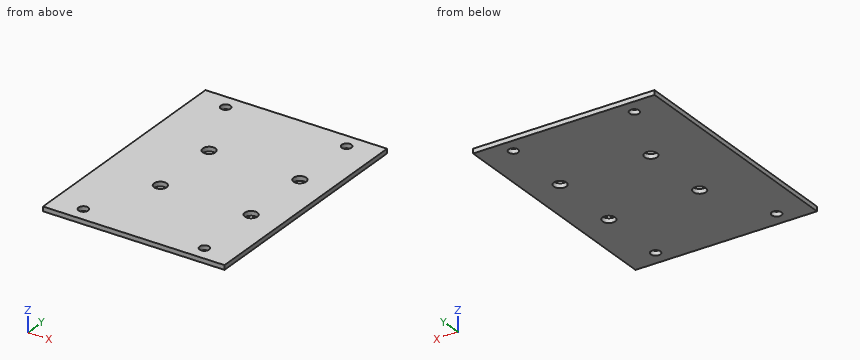
Autodesk Inventor part; units mm, degrees
ref_plane "YZ Plane" through (0, 0, 0) normal (1, 0, 0) x (0, 1, 0)
ref_plane "XZ Plane" through (0, 0, 0) normal (0, 1, 0) x (-1, 0, 0)
ref_plane "XY Plane" through (0, 0, 0) normal (0, 0, 1) x (1, 0, 0)
sketch "スケッチ1" plane through (0, 0, 0) normal (0, 0, 1) x (1, 0, 0)
  line L0 (0, 0) -> (60, 0)
  line L1 (60, 0) -> (60, 80)
  line L2 (60, 80) -> (0, 80)
  line L3 (0, 80) -> (0, 0)
  dimension "d0" = 80
  dimension "d1" = 60
extrude "押し出し1" add sketch "スケッチ1" along normal blind 1.5
sketch "スケッチ2" plane through (0, 0, 1.5) normal (0, 0, 1) x (1, 0, 0)
  line L0 (60, 0) -> (60, 80)
  line L1 (0, 0) -> (60, 0)
  line L2 (60, 80) -> (0, 80)
  point P0 (10, 5)
  point P1 (50, 5)
  point P2 (50, 75)
  point P3 (10, 75)
  dimension "d4" = 10
  dimension "d5" = 40
  dimension "d7" = 5
  dimension "d8" = 5
hole "穴1" at (10, 5, 1.5) at (50, 5, 1.5) at (50, 75, 1.5) at (10, 75, 1.5) direction (0, 0, -1) diameter 3.2 depth 8.8 tip angle 118
sketch "スケッチ3" plane through (0, 0, 1.5) normal (0, 0, 1) x (1, 0, 0)
  line L0 (60, 80) -> (0, 80)
  line L1 (60, 0) -> (60, 80)
  point P0 (0, 0)
  point P1 (20, 52)
  point P2 (50, 52)
  point P3 (50, 28)
  point P4 (20, 28)
  dimension "d16" = 30
  dimension "d17" = 24
  dimension "d18" = 28
  dimension "d19" = 10
hole "穴2" at (20, 52, 1.5) at (50, 52, 1.5) at (50, 28, 1.5) at (20, 28, 1.5) direction (0, 0, -1) diameter 4.2 depth 8.8 tip angle 118
properties part number "キャスター土台"
The model under review builds one solid part; all positions refer to its coordinate system, in mm. Give positions to 0.01 mm unless a question says otherwise; leave off trailing zeros. Order: outer loops, then holes, each group sorted by start corner. A loop starts at its lowest first (then second) coordinate and runs counter-clockwise, first axis right, second up. Notation, with made-up numbers: M 78.25,16.5 L 90.25,16.5 A12 ccw 90.25,37.5 Z; hole C 4,67 d3. An arc over 180 degrees is marked long. Answer in a Markdown table with one row per item. Add a question column.
1. For pin 1 Ø5.5 at (x, y) = (20, 52) entering from -Z; pin 2 Ø4 at (x, y) = (50, 28) entering from -Z, all flat-tipped, find the tip position at first contact; note any pin that passes through.
2. To check wall thickness, follow line 1 along X through (y, z) = (75, 0.75); line 2 along X through (y, z) = (28, 1.1); line 3 along Y through (x, z) = (50, 0.45). State the ranges of each line that lie inside material, in increasing order.
3. Add section B-B on x = 20. State the section outline as (y, z) points, plus the area to 3 significant figures.
4. Add section D-D on x = 50. State the section outline as (y, z) points.
5. Add section C-C on z = 0.3. Count the separate pieces of the cut face and the enclosed holes in it, plus the area to 3 significant figures.
6. Add section A-A on y = 5. State the section outline as (x, z) points, plus the area to 3 significant figures.
The answers:
| question | item | result |
|---|---|---|
| 1 | pin 1 | z = 0 |
| 1 | pin 2 | through |
| 2 | line 1 | 0 to 8.4, 11.6 to 48.4, 51.6 to 60 |
| 2 | line 2 | 0 to 17.9, 22.1 to 47.9, 52.1 to 60 |
| 2 | line 3 | 0 to 3.4, 6.6 to 25.9, 30.1 to 49.9, 54.1 to 73.4, 76.6 to 80 |
| 3 | outline | M 0,0 L 25.9,0 L 25.9,1.5 L 0,1.5 Z; M 30.1,0 L 49.9,0 L 49.9,1.5 L 30.1,1.5 Z; M 54.1,0 L 80,0 L 80,1.5 L 54.1,1.5 Z |
| 3 | area | 107 mm2 |
| 4 | outline | M 0,0 L 3.4,0 L 3.4,1.5 L 0,1.5 Z; M 6.6,0 L 25.9,0 L 25.9,1.5 L 6.6,1.5 Z; M 30.1,0 L 49.9,0 L 49.9,1.5 L 30.1,1.5 Z; M 54.1,0 L 73.4,0 L 73.4,1.5 L 54.1,1.5 Z; M 76.6,0 L 80,0 L 80,1.5 L 76.6,1.5 Z |
| 5 | separate pieces | 1 |
| 5 | enclosed holes | 8 |
| 5 | area | 4,710 mm2 |
| 6 | outline | M 0,0 L 8.4,0 L 8.4,1.5 L 0,1.5 Z; M 11.6,0 L 48.4,0 L 48.4,1.5 L 11.6,1.5 Z; M 51.6,0 L 60,0 L 60,1.5 L 51.6,1.5 Z |
| 6 | area | 80.4 mm2 |
